Input: part model. Units: mm. Frame: model coordinates. A direction names the side the tool comes from. Coordinates: 2 decimals unless noted, no trailing zeros. Write each loop counter-clockwise with the first axis right and the second up, starting at its lowest first coordinate (ties: lowest second). Pieces come first, ordered by that corner, then holes. Notation, with made-up numbers: (41, 55.5) -> (81, 55.5) arc R10 ccw to (81, 72.5) -> close; hole circle Ø1 at (20, 89). An arc over 180 degrees is marked (long way). Use one line per item in the form item = value. Start each with the question number.
(1) Ray query, line 1 along Y through (x, z) = (-8.8, 0); line 2 along Y through (x, z) = (-2.25, 0); line 3 along X through (y, z) = (4.5, 0.25). Return the intervals inside material, ascending.
(2) Cut plane C-C on x = -1. Return the cut outline in (y, z).
(3) First-contact query: pin 1 (2 mm diameter, centred on x = -10, z = 6, fed in from +Y); pin 2 (4.5 mm diameter, centred on y = 0, z = 0, fed in from -X); pin 3 (3 mm diameter, centred on x = -2.5, y = -4, fed in from -Z); pin 4 (1 mm diameter, centred on x = -6.5, y = 6.5, fed in from -Z). Flat tips, straight axial feed; report the tip coordinate or a pass-through.
(4) Set-up query: faces 4 (the face through (-1.01, 7.81, -1.73)), 5 (the face through (0, 0, -3)), 6 (the face through (-9.34, -4.88, -1.08)). Return all of +Z, -Z, +X, -X, +Y, -Y with unobstructed straight access to the full face (end or side cutting, diameter ignored); none if empty.
(5) Cut plane D-D on x = -7. Return the cut outline in (y, z).
(6) Cut plane A-A on y = 0. Return the cut outline in (x, z).
(7) Pull-direction query (Y, two-part tool) for faces 1 (the face through (-3.254, -2.685, 0.596)), 2 (the face through (-6, 0, -10)), 3 (the face through (-12, 5.2, -0.1)); classes: released by +Y, released by -Y, zero draft, split by the parting line, or undercut.
```python
from build123d import *

# Parameters (mm, degrees)
FRONT_CHAMFERS_SIZE        = 2
MOUNTING_SCREW_D           = 5.5
MOUNTING_SCREW_DEPTH       = 12
MOUNTING_SCREW_CBORE_D     = 10
MOUNTING_SCREW_CBORE_DEPTH = 5.4
MOUNTING_SCREW_TIP         = 1.652366702


with BuildPart() as part:
    # Sketch1 → body (revolve)
    with BuildSketch(Plane.XY, mode=Mode.PRIVATE) as body_sk:
        Polygon((0, 0), (0, 8), (-2, 8), (-2, 10), (-12, 10), (-12, 0), align=None)
    revolve(body_sk.sketch.rotate(Axis((0, 0, 0), (1, 0, 0)), 90), axis=Axis((0, 0, 0), (1, 0, 0)))

    # front_chamfers
    front_chamfers_edges = [part.edges().sort_by_distance(p)[0] for p in [
        (-12, 0, -10),
    ]]
    chamfer(front_chamfers_edges, length=FRONT_CHAMFERS_SIZE)

    # mounting_screw
    with Locations(Plane.ZY.offset(12)):
        with Locations((0, 0)):
            CounterBoreHole(MOUNTING_SCREW_D / 2, MOUNTING_SCREW_CBORE_D / 2, MOUNTING_SCREW_CBORE_DEPTH, depth=MOUNTING_SCREW_DEPTH)
            with Locations((0, 0, -(MOUNTING_SCREW_DEPTH + MOUNTING_SCREW_TIP / 2))):  # 118° drill point
                Cone(0, MOUNTING_SCREW_D / 2, MOUNTING_SCREW_TIP, mode=Mode.SUBTRACT)


solid = part.part
```
Values:
q1.line_1 = -10 to -5, 5 to 10
q1.line_2 = -10 to -2.75, 2.75 to 10
q1.line_3 = -6.6 to 0
q2.outline = circle Ø16 at (0, 0); hole circle Ø5.5 at (0, 0)
q3.pin_1 = 8.66
q3.pin_2 = through
q3.pin_3 = -9.68
q3.pin_4 = -8
q4.face_4 = +X
q4.face_5 = +Z, -Z, +X, +Y, -Y
q4.face_6 = -X
q5.outline = circle Ø20 at (0, 0); hole circle Ø10 at (0, 0)
q6.outline = (-12, -8) -> (-10, -10) -> (-2, -10) -> (-2, -8) -> (0, -8) -> (0, -2.75) -> (-6.6, -2.75) -> (-6.6, -5) -> (-12, -5) -> close; (-12, 5) -> (-6.6, 5) -> (-6.6, 2.75) -> (0, 2.75) -> (0, 8) -> (-2, 8) -> (-2, 10) -> (-10, 10) -> (-12, 8) -> close
q7.face_1 = undercut
q7.face_2 = split by the parting line
q7.face_3 = zero draft
